from build123d import *

# Parameters (mm, degrees)
F1_DEPTH = 1
F2_R     = 0.5
F3_DEPTH = 1.001
F4_SIZE  = 0.5
F5_R     = 2
F6_R     = 1.5
F7_DEPTH = 1.001
F8_W     = 5
F8_H     = 6.9
F9_DEPTH = 1.85


with BuildPart() as f1:
    # F0 (on Top) → F1 (new body)
    with BuildSketch(Plane.XY):
        Polygon((17.5, 5), (17.5, 9), (-19, 9), (-19, -9), (17.5, -9), (17.5, -8), (19, -6.5), (19, 3.5), align=None)
    extrude(amount=F1_DEPTH)

    # F2 (on face) → F3 (cut, through all)
    with BuildSketch(Plane.XY.offset(1)):
        with Locations((13.96, -8.25)):
            Circle(F2_R)
        with Locations((11.42, -8.25)):
            Circle(F2_R)
        with Locations((8.88, -8.25)):
            Circle(F2_R)
        with Locations((6.34, -8.25)):
            Circle(F2_R)
        with Locations((3.8, -8.25)):
            Circle(F2_R)
        with Locations((1.26, -8.25)):
            Circle(F2_R)
        with Locations((-1.28, -8.25)):
            Circle(F2_R)
        with Locations((-3.82, -8.25)):
            Circle(F2_R)
        with Locations((-6.36, -8.25)):
            Circle(F2_R)
        with Locations((-8.9, -8.25)):
            Circle(F2_R)
        with Locations((-11.44, -8.25)):
            Circle(F2_R)
        with Locations((-13.98, -8.25)):
            Circle(F2_R)
        with Locations((13.96, 8.25)):
            Circle(F2_R)
        with Locations((11.42, 8.25)):
            Circle(F2_R)
        with Locations((8.88, 8.25)):
            Circle(F2_R)
        with Locations((-1.28, 8.25)):
            Circle(F2_R)
        with Locations((1.26, 8.25)):
            Circle(F2_R)
        with Locations((-6.36, 8.25)):
            Circle(F2_R)
        with Locations((-8.9, 8.25)):
            Circle(F2_R)
        with Locations((-3.82, 8.25)):
            Circle(F2_R)
        with Locations((3.8, 8.25)):
            Circle(F2_R)
        with Locations((6.34, 8.25)):
            Circle(F2_R)
        with Locations((-13.98, 8.25)):
            Circle(F2_R)
        with Locations((-11.44, 8.25)):
            Circle(F2_R)
        with Locations((16.75, 6.46)):
            Circle(F2_R)
        with Locations((16.75, 3.92)):
            Circle(F2_R)
        with Locations((16.75, 1.38)):
            Circle(F2_R)
        with Locations((16.75, -1.16)):
            Circle(F2_R)
        with Locations((16.75, -3.7)):
            Circle(F2_R)
        with Locations((16.75, -6.24)):
            Circle(F2_R)
    extrude(amount=-F3_DEPTH, mode=Mode.SUBTRACT)

    # F4
    f4_edges = [f1.edges().sort_by_distance(p)[0] for p in [
        (17.5, 9, 0.5),
        (17.5, -9, 0.5),
    ]]
    chamfer(f4_edges, length=F4_SIZE)

    # F5
    f5_edges = [f1.edges().sort_by_distance(p)[0] for p in [
        (-19, -9, 0.5),
        (-19, 9, 0.5),
    ]]
    fillet(f5_edges, radius=F5_R)

    # F6 (on face) → F7 (cut, through all)
    with BuildSketch(Plane.XY.offset(1)):
        with Locations((-17, 7)):
            Circle(F6_R)
        with Locations((-17, -7)):
            Circle(F6_R)
    extrude(amount=-F7_DEPTH, mode=Mode.SUBTRACT)

    # F8 (on face) → F9 (join)
    with BuildSketch(Plane.XY.offset(1)):
        with Locations((-16.5, 0)):
            Rectangle(F8_W, F8_H)
    extrude(amount=F9_DEPTH)


solid = f1.part
Input: part model. Units: mm. Frame: model coordinates. A direction names the side the tool comes from. Give positions to 0.01 mm unless a question says otherwise; leave off trailing zeros. Write each loop counter-clockwise with the first axis right and the second up, starting at its lowest first coordinate (ties: lowest second). Pieces come first, ordered by that corner, then holes. Notation, with made-up numbers: (4, -8) -> (48, -8) arc R15 cw to (48, 7) -> close; hole circle Ø4 at (78.25, 79.25). An arc over 180 degrees is marked (long way). Use one line per item in the form item = value. Start each with the question number.
1) Ray query, probe 1 along Y at (x, z) = (-3.82, 0.8); probe 2 along Y at (x, z) = (-17, 0.4); probe 3 along X at (y, z) = (0.25, 1.5). Return the intervals inside material, ascending. Write a range as from..to.
2) Section query A-A on y = -1.16. Return the cut outline in (x, z), then the cut area to 4 significant figures.
3) Draft query along X for faces 3 (the cylindrical face through (-3.928, -8.738, 0.507)), 4 (the flat face through (-19, 0, 1)), 5 (the flat face through (17.5, 6.7, 0.5)). Return one class per face: pulls with the +X half, pulls with the -X half, needs draft (parallel to the pull), parting line crosses it, or undercut.
4) Set-up query: faces 1 (the flat face through (-14, 0, 2)), 2 (the cylindrical face through (-1.049, -8.694, 0.507)). Return all of +Z, -Z, +X, -X, +Y, -Y with unobstructed straight access to the full face (end or side cutting, diameter ignored); none if empty.
5) Section query B-B on x = -6.36. Return the cut outline in (y, z).
6) Section query D-D on z = 1.8. Return the cut outline in (x, y), then the cut area to 3 significant figures.
7) Pin query (flat end, axial travel): pin 1 (0.9 mm diameter, centred on y = 0, z = 2, fed in from +X); pin 2 (3.5 mm diameter, centred on x = -17, y = -7, fed in from +Z); pin 3 (1.5 mm diameter, centred on x = -16, z = 1.5, fed in from -Y); pin 4 (0.6 mm diameter, centred on x = -17, z = 2, fed in from +Y). Return the tip coordinate at first contact, or that it passes through.
8) Section query C-C on x = -12.5. Return the cut outline in (y, z).
Outcome:
q1.probe_1 = -9..-8.75, -7.75..7.75, 8.75..9
q1.probe_2 = -9..-8.5, -5.5..5.5, 8.5..9
q1.probe_3 = -19..-14
q2.outline = (-19, 0) -> (16.25, 0) -> (16.25, 1) -> (-14, 1) -> (-14, 2.85) -> (-19, 2.85) -> close; (17.25, 0) -> (19, 0) -> (19, 1) -> (17.25, 1) -> close
q2.area = 46.25 mm^2
q3.face_3 = undercut
q3.face_4 = pulls with the -X half
q3.face_5 = pulls with the +X half
q4.face_1 = +Z, +X, +Y, -Y
q4.face_2 = +Z, -Z
q5.outline = (-9, 0) -> (-8.75, 0) -> (-8.75, 1) -> (-9, 1) -> close; (-7.75, 0) -> (7.75, 0) -> (7.75, 1) -> (-7.75, 1) -> close; (8.75, 0) -> (9, 0) -> (9, 1) -> (8.75, 1) -> close
q6.outline = (-19, -3.45) -> (-14, -3.45) -> (-14, 3.45) -> (-19, 3.45) -> close
q6.area = 34.5 mm^2
q7.pin_1 = -14
q7.pin_2 = 1
q7.pin_3 = -9
q7.pin_4 = 3.45
q8.outline = (-9, 0) -> (9, 0) -> (9, 1) -> (-9, 1) -> close
